Autodesk Inventor part; units mm, degrees
ref_plane "YZ Plane" through (0, 0, 0) normal (1, 0, 0) x (0, 1, 0)
ref_plane "XZ Plane" through (0, 0, 0) normal (0, 1, 0) x (-1, 0, 0)
ref_plane "XY Plane" through (0, 0, 0) normal (0, 0, 1) x (1, 0, 0)
sketch "Sketch1" plane through (0, 0, 0) normal (0, 1, 0) x (-1, 0, 0)
  line L0 (25.4, 25.4) -> (-25.4, 25.4)
  line L1 (-25.4, 25.4) -> (-25.4, -25.4)
  line L2 (-25.4, -25.4) -> (25.4, -25.4)
  line L3 (25.4, -25.4) -> (25.4, 25.4)
  line L4 (25.4, 25.4) -> (-25.4, -25.4) construction
  line L5 (-25.4, 25.4) -> (25.4, -25.4) construction
  point P0 (0, 0)
  dimension "d0" = 50.8
  dimension "d1" = 50.8
extrude "Extrusion1" add sketch "Sketch1" along normal blind 5.08
sketch "Sketch2" plane through (0, 5.08, 0) normal (0, 1, 0) x (1, 0, 0)
  line L0 (-25.4, -25.4) -> (25.4, -25.4)
  line L1 (-25.4, 25.4) -> (-25.4, -25.4)
  line L2 (25.4, -25.4) -> (25.4, 25.4)
  line L3 (25.4, 25.4) -> (-25.4, 25.4)
  point P0 (0, 0)
  point P1 (-19.05, -19.05)
  point P2 (-19.05, 19.05)
  point P3 (19.05, 19.05)
  point P4 (19.05, -19.05)
  dimension "d4" = 6.35
  dimension "d5" = 6.35
  dimension "d6" = 6.35
  dimension "d7" = 6.35
  dimension "d8" = 6.35
  dimension "d9" = 6.35
  dimension "d10" = 6.35
  dimension "d11" = 6.35
hole "Hole1" at (-19.05, 5.08, 19.05) at (19.05, 5.08, 19.05) at (19.05, 5.08, -19.05) at (-19.05, 5.08, -19.05) direction (0, -1, 0) diameter 3.937 end through all counterbore diameter 9.525 counterbore depth 2.54
sketch "Sketch3" plane through (0, 0, 0) normal (0, -1, 0) x (1, 0, 0)
  line L0 (-29.21, -25.4) -> (-29.21, 25.4)
  line L1 (-25.4, 25.4) -> (-25.4, -25.4)
  line L2 (-25.4, -25.4) -> (25.4, -25.4)
  line L3 (29.21, -25.4) -> (29.21, -29.21)
  line L4 (29.21, -29.21) -> (-29.21, -29.21)
  line L5 (-29.21, -29.21) -> (-29.21, -25.4)
  line L6 (25.4, -25.4) -> (-25.4, -25.4)
  line L7 (29.21, -25.4) -> (29.21, 25.4)
  line L8 (25.4, 25.4) -> (25.4, -25.4)
  line L9 (-25.4, 25.4) -> (25.4, 25.4)
  line L10 (29.21, 25.4) -> (29.21, 29.21)
  line L11 (29.21, 29.21) -> (-29.21, 29.21)
  line L12 (-29.21, 29.21) -> (-29.21, 25.4)
  point P0 (0, 0)
  dimension "d20" = 58.42
  dimension "d21" = 3.81
  dimension "d23" = 58.42
  dimension "d24" = 3.81
extrude "Extrusion2" add sketch "Sketch3" against normal blind 88.9
fillet "Fillet1" radius 3.175 1 edges at (29.21, 44.45, -29.21)
sketch "Sketch4" plane through (-29.21, 0, -26.035) normal (-1, 0, 0) x (0, 0, 1)
  line L0 (13.335, 83.82) -> (38.735, 83.82)
  line L1 (38.735, 83.82) -> (38.735, 80.01)
  line L2 (38.735, 80.01) -> (13.335, 80.01)
  line L3 (13.335, 80.01) -> (13.335, 83.82)
  line L4 (0, 88.9) -> (52.07, 88.9)
  line L5 (55.245, 0) -> (55.245, 88.9)
  line L6 (-3.175, 88.9) -> (-3.175, 0)
  point P0 (26.035, 0)
  dimension "d28" = 25.4
  dimension "d29" = 5.08
  dimension "d30" = 3.81
  dimension "d31" = 16.51
  dimension "d32" = 16.51
extrude "Extrusion3" cut sketch "Sketch4" against normal through all
properties part number "vertical batter holder 4 holes in bottom"
Model file for the job. Use its own axes, mm. A direction names the side the tool comes from. Coordinates: 2 decimals unless noted, no trailing zeros. Order: outer loops, then holes, each group sorted by start corner. A loop starts at its lowest first (then second) coordinate and runs counter-clockwise, first axis right, second up. Notation, with made-up numbers: (50, 58.25) -> (75, 58.25) arc R30 cw to (75, 86.25) -> close; hole circle Ø6 at (56.5, 58.25). An arc over 180 degrees is marked (long way). Return JSON: item names as keys, results as strings.
Item 1: Slice it at B-B (y = 19). Write the cut outline in (x, z) (3 decimals).
Model answer:
{"outline": "(-29.21, -29.21) -> (26.035, -29.21) arc R3.175 ccw to (29.21, -26.035) -> (29.21, 29.21) -> (-29.21, 29.21) -> close; hole (-25.4, -25.4) -> (25.4, -25.4) -> (25.4, 25.4) -> (-25.4, 25.4) -> close"}
Item 2: Pin check, flat tips, straight feed: P1, Ø2, axis at x = -20.5, z = 0, coming from the +Y side; P2, Ø3, axis at x = -19, z = 17, coming from the +Y side. Stop position of each tip, or through.
Model answer:
{"P1": "stops at y = 5.08", "P2": "stops at y = 2.54"}
Item 3: 3-axis set-ups, long thin cutter, end or side, ignore diameter. For faces 1 (the face through (0, 46, 25.4)), 2 (the face through (18.46, 1.25, 20.93)), 3 (the face through (-27, 80.01, 0)): which of +Z, -Z, +X, -X, +Y, -Y reach the whole face in a straight line?
Model answer:
{"face 1": "+Y", "face 2": "+Y, -Y", "face 3": "+X, -X"}
Item 4: Slice it at A-A (z = -1.5). Write the cut outline in (x, y).
Model answer:
{"outline": "(-29.21, 0) -> (29.21, 0) -> (29.21, 80.01) -> (25.4, 80.01) -> (25.4, 5.08) -> (-25.4, 5.08) -> (-25.4, 80.01) -> (-29.21, 80.01) -> close; (-29.21, 83.82) -> (-25.4, 83.82) -> (-25.4, 88.9) -> (-29.21, 88.9) -> close; (25.4, 83.82) -> (29.21, 83.82) -> (29.21, 88.9) -> (25.4, 88.9) -> close"}
Item 5: Slice it at D-D (x = -12.5). Write the cut outline in (y, z).
Model answer:
{"outline": "(0, -29.21) -> (88.9, -29.21) -> (88.9, -25.4) -> (5.08, -25.4) -> (5.08, 25.4) -> (88.9, 25.4) -> (88.9, 29.21) -> (0, 29.21) -> close"}
Item 6: Mould opens along Z. For faces 4 (the face through (-1, 44, -29.21)), 5 (the face through (0, 44, 29.21)), 6 (the face through (17.72, 1.25, -20.5)), 7 (the face through (27, 82, 12.7)) say: pulls with the +Z half, pulls with the -Z half, needs draft (parallel to the pull), parting line crosses it, or undercut.
Model answer:
{"face 4": "pulls with the -Z half", "face 5": "pulls with the +Z half", "face 6": "undercut", "face 7": "undercut"}
Item 7: Slice it at C-C (x = -19.05). Write the cut outline in (y, z), then the cut area to 3 significant figures.
Model answer:
{"outline": "(0, -29.21) -> (88.9, -29.21) -> (88.9, -25.4) -> (5.08, -25.4) -> (5.08, -23.81) -> (2.54, -23.81) -> (2.54, -21.02) -> (0, -21.02) -> close; (0, -17.08) -> (2.54, -17.08) -> (2.54, -14.29) -> (5.08, -14.29) -> (5.08, 14.29) -> (2.54, 14.29) -> (2.54, 17.08) -> (0, 17.08) -> close; (0, 21.02) -> (2.54, 21.02) -> (2.54, 23.81) -> (5.08, 23.81) -> (5.08, 25.4) -> (88.9, 25.4) -> (88.9, 29.21) -> (0, 29.21) -> close", "area": "867 mm²"}
Item 8: Wall check: line 1 along Z through (x, y) = (19.05, 4.25); line 2 along X through (y, z) = (0.8, -19.05). Give the ranges that are in metal, low to high. Write a range as from..to.
Model answer:
{"line 1": "z = -29.21..-23.81, -14.29..14.29, 23.81..29.21", "line 2": "x = -29.21..-21.02, -17.08..17.08, 21.02..29.21"}
